Source: three-view drawing plus pictorial views. Frame: mm from the lowest corner of the part. Coordinates: 2 decimals unless noted, no trailing zeros. Loops run counter-clockwise (first coordinate to the right, second up) from the corner with the lowest first, then second, coordinate; pieces in that order, holes last. Notation, with made-up numbers: M 48,13.5 L 98,13.5 A24 ccw 98,51.5 Z; hole C 1,35.5 d6. An arc over 180 degrees is marked long. Use a Markdown table: item, result. Add a question column.
1. Line query: L1, parallel to Z at x = 18.5, y = 4.45; L2, parallel to X at y = 1.9, z = 7 (1 decimal); L3, parallel to Z at x = 7, y = 0.35. Output: solid intervals per line, ascending. Write a range as [from, to].
2. Section B-B on x = 24. Output: boundary loops of the cut face in (y, z).
3. Section D-D on y = 0.75. Output: boundary loops of the cut face in (x, z), then the cut area to 3 significant figures.
4. Pin query (flat end, axial travel): pin 1 (1.2 mm diameter, centred on y = 1.5, z = 21.5, fed in from +X); pin 2 (0.8 mm diameter, centred on y = 1.5, z = 25.5, fed in from -X); pin 3 (1.9 mm diameter, centred on x = 6.16, z = 6.16, fed in from -Y); pin 4 (2 mm diameter, centred on x = 36, y = 2.5, fed in from -Z). Return the tip coordinate at first contact, or that it passes through.
5. Section A-A on z = 18.5. Output: boundary loops of the cut face in (x, y).
6. Section C-C on y = 3.05. Output: boundary loops of the cut face in (x, z), then the cut area to 3 significant figures.
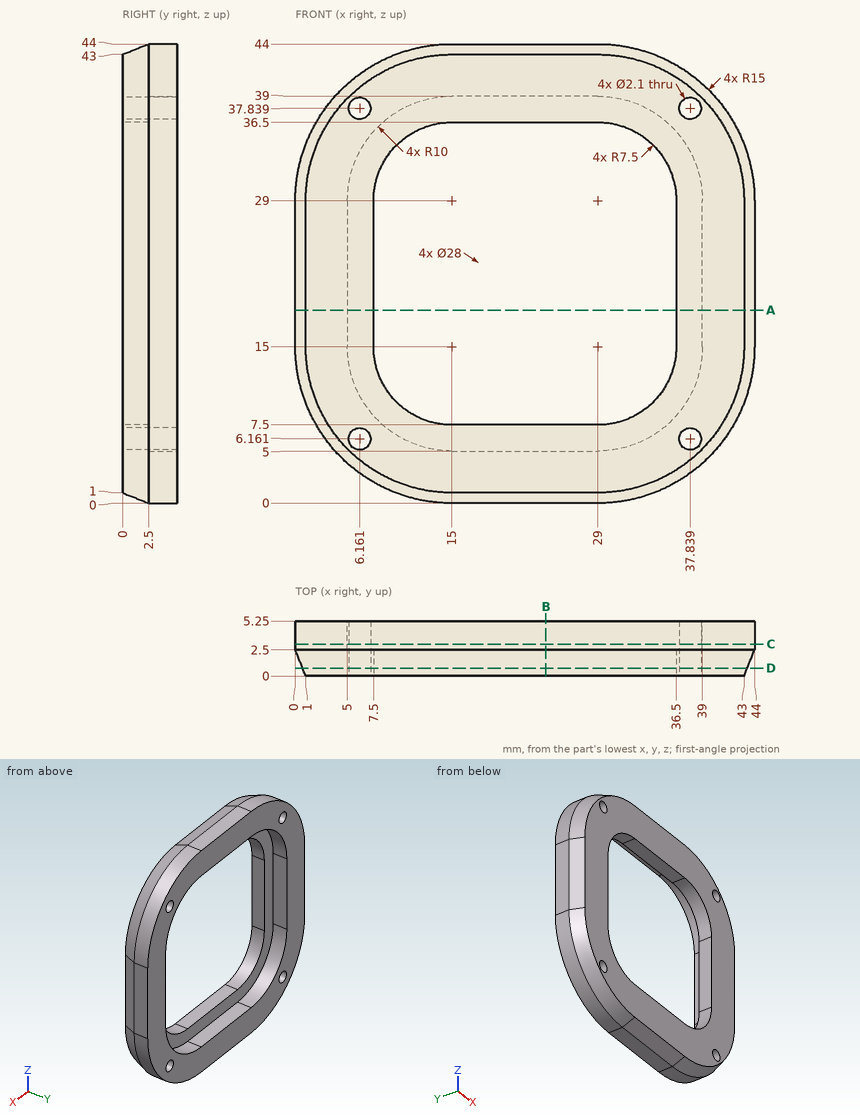
Answers below:
| question | item | result |
|---|---|---|
| 1 | L1 | z = [0, 5], [39, 44] |
| 1 | L2 | x = [2.6, 5.5], [6.8, 37.2], [38.5, 41.4] |
| 1 | L3 | z = [3.34, 5.53], [6.79, 37.21], [38.47, 40.66] |
| 2 | outline | M 0,1 L 2.5,0 L 5.25,0 L 5.25,5 L 2.5,5 L 2.5,7.5 L 0,7.5 Z; M 0,36.5 L 2.5,36.5 L 2.5,39 L 5.25,39 L 5.25,44 L 2.5,44 L 0,43 Z |
| 3 | outline | M 0.7,15 A14.3 ccw 15,0.7 L 29,0.7 A14.3 ccw 43.3,15 L 43.3,29 A14.3 ccw 29,43.3 L 15,43.3 A14.3 ccw 0.7,29 Z; hole C 6.16,6.16 d2.1; hole C 6.16,37.84 d2.1; hole M 7.5,15 A7.5 ccw 15,7.5 L 29,7.5 A7.5 ccw 36.5,15 L 36.5,29 A7.5 ccw 29,36.5 L 15,36.5 A7.5 ccw 7.5,29 Z; hole C 37.84,6.16 d2.1; hole C 37.84,37.84 d2.1 |
| 3 | area | 833 mm² |
| 4 | pin 1 | stops at x = 43.84 |
| 4 | pin 2 | stops at x = 0.24 |
| 4 | pin 3 | passes through |
| 4 | pin 4 | stops at z = 1.25 |
| 5 | outline | M 0,2.5 L 1,0 L 7.5,0 L 7.5,2.5 L 5,2.5 L 5,5.25 L 0,5.25 Z; M 36.5,0 L 43,0 L 44,2.5 L 44,5.25 L 39,5.25 L 39,2.5 L 36.5,2.5 Z |
| 6 | outline | M 0,15 A15 ccw 15,0 L 29,0 A15 ccw 44,15 L 44,29 A15 ccw 29,44 L 15,44 A15 ccw 0,29 Z; hole M 5,15 A10 ccw 15,5 L 29,5 A10 ccw 39,15 L 39,29 A10 ccw 29,39 L 15,39 A10 ccw 5,29 Z; hole C 6.16,6.16 d2.1; hole C 6.16,37.84 d2.1; hole C 37.84,6.16 d2.1; hole C 37.84,37.84 d2.1 |
| 6 | area | 659 mm² |
